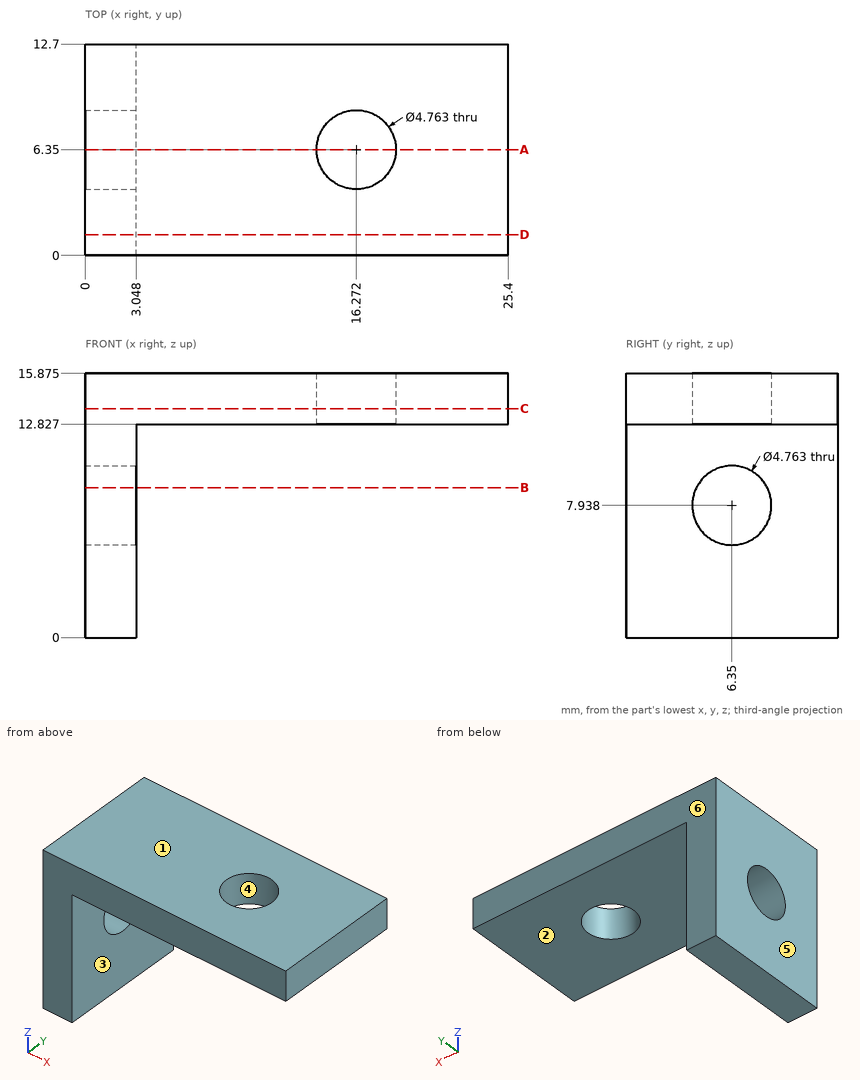
For this review, use the dimensioned drawing (mm, ordinates from the lowest corner) and the shaded views. A direction names the side the tool comes from. Coordinates: 2 decimals unless noted, no trailing zeros. Loops run counter-clockwise (first coordinate to the right, second up) from the corner with the lowest first, then second, coordinate; pieces in that order, holes last. Notation, with made-up numbers: (-38.75, 72) -> (-23.75, 72) arc R17 cw to (-23.75, 76) -> close; hole circle Ø5 at (88, 58.5). An arc over 180 degrees is marked (long way). Use a Markdown table: item, result. Add a question column.
Item 1: We need section A-A, the plane y = 6.35. Write out the cut boundary in (x, z) (1 decimal).
Item 2: Wall thickness on L1, parallel to X at y = 10.25, z = 11.75; L2, parallel to Z at x = 10, y = 10.75 (1 decimal); L3, parallel to Y at x = 2.5, z = 6.5: over which ranges is each line inside the solid? List them lowest first. Write a range as from..to.
Item 3: We need section B-B, the plane z = 9. Write out the cut boundary in (x, y), and give its area (3 significant figures).
Item 4: Machinability: for the marked faces 1 and 2, which of the approach directions +Z, -Z, +X, -X, +Y, -Y give a long, thin tool a straight path to every point of the face, cutting with its end or side? Answer none if there is none.
Item 5: Clearance check with flat-ended pins moving along their axes: P1, Ø6, axis at y = 6.35, z = 7.94, coming from the +X side; P2, Ø2, axis at y = 9.5, z = 6, coming from the -X side; P3, Ø4, axis at x = 11, y = 8, coming from the -Z side. State where each tip first meets the part, or that it passes through.
Item 6: The part is to be moulded in two halves that separate along X. For the marked faces 3, 4, 5 and 6, say which applies: +X half, -X half, draft (parallel to the pull), parting line (faces both ways), or undercut.
Item 7: We need section C-C, the plane z = 13.75. Write out the cut boundary in (x, y), and give its area (3 significant figures).
Item 8: We need section D-D, the plane y = 1.25. Write out the cut boundary in (x, z) (1 decimal).
Numbers:
| question | item | result |
|---|---|---|
| 1 | outline | (0, 0) -> (3, 0) -> (3, 5.6) -> (0, 5.6) -> close; (0, 10.3) -> (3, 10.3) -> (3, 12.8) -> (13.9, 12.8) -> (13.9, 15.9) -> (0, 15.9) -> close; (18.7, 12.8) -> (25.4, 12.8) -> (25.4, 15.9) -> (18.7, 15.9) -> close |
| 2 | L1 | x = 0..3.05 |
| 2 | L2 | z = 12.8..15.9 |
| 2 | L3 | y = 0..4.45, 8.25..12.7 |
| 3 | outline | (0, 0) -> (3.05, 0) -> (3.05, 4.22) -> (0, 4.22) -> close; (0, 8.48) -> (3.05, 8.48) -> (3.05, 12.7) -> (0, 12.7) -> close |
| 3 | area | 25.7 mm^2 |
| 4 | face 1 | +Z, +X, -X, +Y, -Y |
| 4 | face 2 | -Z, +X, +Y, -Y |
| 5 | P1 | stops at x = 3.05 |
| 5 | P2 | stops at x = 0 |
| 5 | P3 | stops at z = 12.83 |
| 6 | face 3 | +X half |
| 6 | face 4 | undercut |
| 6 | face 5 | -X half |
| 6 | face 6 | draft |
| 7 | outline | (0, 0) -> (25.4, 0) -> (25.4, 12.7) -> (0, 12.7) -> close; hole circle Ø4.76 at (16.27, 6.35) |
| 7 | area | 305 mm^2 |
| 8 | outline | (0, 0) -> (3, 0) -> (3, 12.8) -> (25.4, 12.8) -> (25.4, 15.9) -> (0, 15.9) -> close |
